```python
from build123d import *

# Parameters (mm, degrees)
F0_R     = 147.5
F0_R_2   = 97.5
F1_DEPTH = 25
F0_R_3   = 90
F2_DEPTH = 50.5
F4_R     = 97.5
F4_R_2   = 7.25
F4_R_3   = 31
F5_DEPTH = 20


with BuildPart() as f1:
    # F0 (on Right) → F1 (new body)
    with BuildSketch(Plane.YZ):
        Circle(F0_R)
        Circle(F0_R_2, mode=Mode.SUBTRACT)
    extrude(amount=F1_DEPTH)

    # F0 (on Right) → F2 (join)
    with BuildSketch(Plane.YZ):
        Circle(F0_R_2)
        Circle(F0_R_3, mode=Mode.SUBTRACT)
    extrude(amount=F2_DEPTH)

    # F4 (on offset) → F5 (join)
    with BuildSketch(Plane.YZ.offset(50.5)):
        Circle(F4_R)
        with Locations((-33.591927, -46.235321)):
            Circle(F4_R_2, mode=Mode.SUBTRACT)
        with Locations((33.591927, -46.235321)):
            Circle(F4_R_2, mode=Mode.SUBTRACT)
        with Locations((-54.35288, 17.660321)):
            Circle(F4_R_2, mode=Mode.SUBTRACT)
        Circle(F4_R_3, mode=Mode.SUBTRACT)
        with Locations((54.35288, 17.660321)):
            Circle(F4_R_2, mode=Mode.SUBTRACT)
        with Locations((0, 57.15)):
            Circle(F4_R_2, mode=Mode.SUBTRACT)
    extrude(amount=F5_DEPTH)


solid = f1.part
```
Input: part model. Units: mm. Frame: model coordinates. A direction names the side the tool comes from. Give positions to 0.01 mm unless a question says otherwise; leave off trailing zeros. Write each loop counter-clockwise with the first axis right and the second up, starting at its lowest first coordinate (ties: lowest second). Pieces come first, ordered by that corner, then holes. Notation, with made-up numbers: (-1.5, -24.5) - (19.5, -24.5) arc R14 ccw to (19.5, -20.5) - close; hole circle Ø11 at (32.25, -27). An arc over 180 degrees is marked (long way). Write item = value, one per line. Start each with the question number.
1) Draft query along Z for faces 4 (the face through (12.32, -31.98, -143.99)), 5 (the face through (25, 31, -96)), 6 (the face through (60.36, -0.94, 64.34)). Return one class per face: pulls with the +Z half, pulls with the -Z half, needs draft (parallel to the pull), parting line crosses it, or undercut.
2) Cut plane D-D (x = 64). Return loops of the section in (y, z).
3) Pin query (flat end, axial travel): pin 1 (23 mm diameter, centred on y = 33.59, z = -46.24, fed in from -X); pin 2 (10 mm diameter, centred on y = 52, z = 98, fed in from +X); pin 3 (2 mm diameter, centred on x = 14, z = 65, fed in from +Y). Return the tip coordinate at first contact, or that it passes through.
4) Cut plane B-B (y = 16.5). Return loops of the section in (x, z).
5) Material intervals for L1, parallel to Z at x = 58, y = 0; L2, parallel to X at y = -9.5, z = 100.5; L3, parallel to X at y = -10.5, z = -77, sorted ascending. Write a range as [from, to].
6) Reachability of faces 1 (the face through (0, -68, -63)), 2 (the face through (47.43, -77.37, -59.33)), 3 (the face through (50.5, -1, -39)) from +Z, -Z, +X, -X, +Y, -Y: full face, straight path, thin tool, end or side. Return the list, or none.
7) Cut plane C-C (x = 34.5). Return loops of the section in (y, z).
8) Cut plane A-A (z = 0). Return loops of the section in (x, y), and give its area (3 significant figures).
Answers follow:
q1.face_4 = parting line crosses it
q1.face_5 = needs draft
q1.face_6 = undercut
q2.outline = circle Ø195 at (0, 0); hole circle Ø14.5 at (-54.35, 17.66); hole circle Ø14.5 at (-33.59, -46.24); hole circle Ø62 at (0, 0); hole circle Ø14.5 at (0, 57.15); hole circle Ø14.5 at (33.59, -46.24); hole circle Ø14.5 at (54.35, 17.66)
q3.pin_1 = 50.5
q3.pin_2 = 25
q3.pin_3 = 132.89
q4.outline = (0, -146.57) - (25, -146.57) - (25, -96.09) - (70.5, -96.09) - (70.5, -26.24) - (50.5, -26.24) - (50.5, -88.47) - (0, -88.47) - close; (0, 88.47) - (50.5, 88.47) - (50.5, 26.24) - (70.5, 26.24) - (70.5, 96.09) - (25, 96.09) - (25, 146.57) - (0, 146.57) - close
q5.L1 = [-97.5, -31], [31, 49.9], [64.4, 97.5]
q5.L2 = [0, 25]
q5.L3 = [50.5, 70.5]
q6.face_1 = +Z, -Z, -X, +Y, -Y
q6.face_2 = +X
q6.face_3 = -X
q7.outline = circle Ø195 at (0, 0); hole circle Ø180 at (0, 0)
q8.outline = (0, -147.5) - (25, -147.5) - (25, -97.5) - (70.5, -97.5) - (70.5, -31) - (50.5, -31) - (50.5, -90) - (0, -90) - close; (0, 90) - (50.5, 90) - (50.5, 31) - (70.5, 31) - (70.5, 97.5) - (25, 97.5) - (25, 147.5) - (0, 147.5) - close
q8.area = 5,920 mm^2
